```python
from build123d import *

# Parameters (mm, degrees)
SKETCH1_R           = 36.11499
BOSS_EXTRUDE1_DEPTH = 3.175
SKETCH2_R           = 9.525
BOSS_EXTRUDE3_DEPTH = 19.05
CHAMFER1_SIZE       = 4.7625
SKETCH5_R           = 15.875
BOSS_EXTRUDE4_DEPTH = 11.90625
BOSS_EXTRUDE5_DEPTH = 14.2875
CIRPATTERN1_COUNT   = 3
BOSS_EXTRUDE6_DEPTH = 14.2875
CIRPATTERN2_COUNT   = 6
SKETCH9_R           = 13.335
CUT_EXTRUDE1_DEPTH  = 11.90625
CHAMFER2_SIZE       = 0.762
CHAMFER3_SIZE       = 0.762


with BuildPart() as part:
    # Sketch1 → Boss-Extrude1 (new body)
    with BuildSketch(Plane(origin=(0, 0, 0), x_dir=(1, 0, 0), z_dir=(0, 1, 0))):
        with Locations(Location((0, 0, 0), (0, 0, 270))):
            Circle(SKETCH1_R)
    extrude(amount=BOSS_EXTRUDE1_DEPTH)

    # Sketch2 → Boss-Extrude3 (add)
    with BuildSketch(Plane(origin=(0, 3.175, 0), x_dir=(1, 0, 0), z_dir=(0, 1, 0))):
        with Locations(Location((0, 0, 0), (0, 0, 90))):
            Circle(SKETCH2_R)
    extrude(amount=BOSS_EXTRUDE3_DEPTH)

    # Chamfer1
    chamfer1_edges = [part.edges().sort_by_distance(p)[0] for p in [
        (0, 22.225, 9.525),
    ]]
    chamfer(chamfer1_edges, length=CHAMFER1_SIZE)

    # Sketch5 → Boss-Extrude4 (add)
    with BuildSketch(Plane.XZ):
        with Locations(Location((0, 0, 0), (0, 0, 270))):
            Circle(SKETCH5_R)
    extrude(amount=BOSS_EXTRUDE4_DEPTH)

    # Sketch6 → Boss-Extrude5 (add)
    with BuildSketch(Plane(origin=(0, 3.175, 0), x_dir=(1, 0, 0), z_dir=(0, 1, 0))):
        with BuildLine():
            Line((-1.5875, 36.080082406), (-1.5875, 9.391776656))
            ThreePointArc((-1.5875, 9.391776656), (0, 9.525), (1.5875, 9.391776656))
            Line((1.5875, 9.391776656), (1.5875, 33.101016708))
            ThreePointArc((1.5875, 33.101016708), (13.411669734, 30.303870682), (23.432855816, 23.432855816))
            Line((23.432855816, 23.432855816), (25.537154331, 25.537154331))
            ThreePointArc((25.537154331, 25.537154331), (13.083761644, 33.661664902), (-1.5875, 36.080082406))
        make_face()
    boss_extrude5 = extrude(amount=BOSS_EXTRUDE5_DEPTH)

    # CirPattern1: Boss-Extrude5 ×3 about axis
    cirpattern1_axis = Axis((0, 22.225, 0), (0, -1, 0))
    for i in range(1, CIRPATTERN1_COUNT):
        add(boss_extrude5.rotate(cirpattern1_axis, i * 360 / CIRPATTERN1_COUNT))

    # Sketch8 → Boss-Extrude6 (add)
    with BuildSketch(Plane(origin=(0, 3.175, 0), x_dir=(1, 0, 0), z_dir=(0, 1, 0))):
        with BuildLine():
            ThreePointArc((14.375330432, 18.734295362), (20.450378012, 11.80703125), (23.412040922, 3.082253661))
            Line((23.412040922, 3.082253661), (26.559878357, 3.496674321))
            ThreePointArc((26.559878357, 3.496674321), (23.200008669, 13.39453125), (16.308147969, 21.253192218))
            Line((16.308147969, 21.253192218), (14.375330432, 18.734295362))
        make_face()
    boss_extrude6 = extrude(amount=BOSS_EXTRUDE6_DEPTH)

    # CirPattern2: Boss-Extrude6 ×6 about axis
    cirpattern2_axis = Axis((0, 0, 0), (0, 1, 0))
    for i in range(1, CIRPATTERN2_COUNT):
        add(boss_extrude6.rotate(cirpattern2_axis, i * 360 / CIRPATTERN2_COUNT))

    # Sketch9 → Cut-Extrude1 (cut)
    with BuildSketch(Plane.XZ.offset(11.90625)):
        with Locations(Location((0, 0, 0), (0, 0, 270))):
            Circle(SKETCH9_R)
    extrude(amount=-CUT_EXTRUDE1_DEPTH, mode=Mode.SUBTRACT)

    # Chamfer2
    chamfer2_edges = [part.edges().sort_by_distance(p)[0] for p in [
        (0, 0, -36.11499),
    ]]
    chamfer(chamfer2_edges, length=CHAMFER2_SIZE)

    # Chamfer3
    chamfer3_edges = [part.edges().sort_by_distance(p)[0] for p in [
        (0, -11.90625, 15.875),
    ]]
    chamfer(chamfer3_edges, length=CHAMFER3_SIZE)


solid = part.part
```
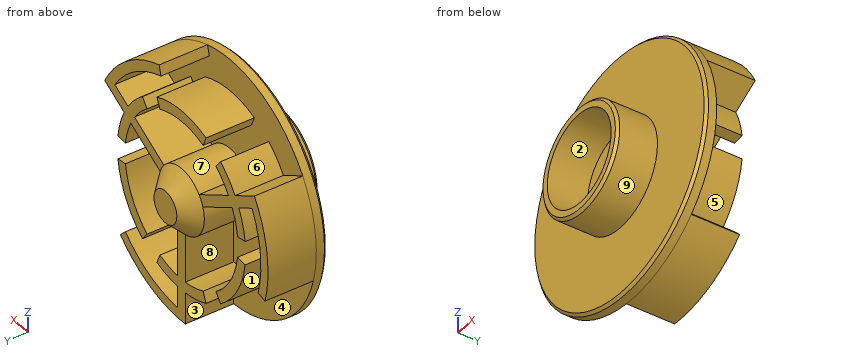
CAD build for the part. Positions are in the model's coordinates, mm. Face numbers are marked on the shaded views. A direction names the side the tool comes from. Round coordinates to 2 decimals unless told otherwise and drop trailing zeros. Order: outer loops, then holes, each group sorted by start corner. A loop starts at its lowest first (then second) coordinate and runs counter-clockwise, first axis right, second up.
Q1. Slice it at B-B (z = 0). Write the cut outline in (x, y) (1 decimal), and give its area (3 significant figures).
Q2. Which spindle directions (+Z, -Z, +X, -X, +Y, -Y) get a long thin tool onto all of the face, cutting with end or side? Do the marked faces 1, 2, 3, 4 and 5. Say none if no direction does.
Q3. Two-plate mould, pull along Z, no slides. Class the marked faces 6, 7, 8 and 9: pulls with the +Z half, pulls with the -Z half, needs draft (parallel to the pull), parting line crosses it, or undercut.
Q4. Slice it at C-C (y = 5). State how many separate pieces and enclosed holes the cut face has, and give its area (3 significant figures).
Q5. Drop flat-ended pins along their axis: pin 1 (8 mm diameter, centred on x = -10, z = -18, fed in from +Y); pin 2 (4.5 mm diameter, centred on y = 13, z = -33, fed in from -X); pin 3 (8 mm diameter, centred on y = -7.5, z = 26.5, fed in from +X); pin 4 (1.5 mm diameter, centred on y = 15, z = 5.5, fed in from -X). Give the stop position or say it passes through.
Q6. Slice it at A-A (x = 0). Write the cut outline in (y, z) (1 decimal).
Q7. Wall check: L1, parallel to X at y = -3.5, z = 0 (3 decimals); L2, parallel to X at y = 6.5, z = -6.5; L3, parallel to Z at x = 15.5, y = 8.5 (3 decimals). Give the ranges that are in metal, low to high.
Results below:
1. outline: (-36.1, 0.8) - (-35.4, 0) - (-15.9, 0) - (-15.9, -11.1) - (-15.1, -11.9) - (-13.3, -11.9) - (-13.3, 0) - (13.3, 0) - (13.3, -11.9) - (15.1, -11.9) - (15.9, -11.1) - (15.9, 0) - (35.4, 0) - (36.1, 0.8) - (36.1, 3.2) - (9.5, 3.2) - (9.5, 17.5) - (4.8, 22.2) - (-4.8, 22.2) - (-9.5, 17.5) - (-9.5, 3.2) - (-33.1, 3.2) - (-33.1, 17.5) - (-36.1, 17.5) - close
1. area: 671 mm2
2. face 1: -Z, +Y
2. face 2: -Y
2. face 3: -Z, -X, +Y
2. face 4: +Y
2. face 5: +X, +Y
3. face 6: pulls with the +Z half
3. face 7: undercut
3. face 8: undercut
3. face 9: parting line crosses it
4. separate pieces: 4
4. enclosed holes: 0
4. area: 1,110 mm2
5. pin 1: stops at y = 17.46
5. pin 2: stops at x = -1.59
5. pin 3: passes through
5. pin 4: stops at x = -35.8
6. outline: (-11.9, -15.1) - (-11.1, -15.9) - (0, -15.9) - (0, -35.4) - (0.8, -36.1) - (17.5, -36.1) - (17.5, -9.5) - (22.2, -4.8) - (22.2, 4.8) - (17.5, 9.5) - (3.2, 9.5) - (3.2, 23.6) - (17.5, 23.6) - (17.5, 26.8) - (3.2, 26.8) - (3.2, 36.1) - (0.8, 36.1) - (0, 35.4) - (0, 15.9) - (-11.1, 15.9) - (-11.9, 15.1) - (-11.9, 13.3) - (0, 13.3) - (0, -13.3) - (-11.9, -13.3) - close
7. L1: x = -15.875 to -13.335, 13.335 to 15.875
7. L2: x = -35.53 to -32.5, -25.99 to -22.7, -6.96 to 6.96, 22.7 to 25.99
7. L3: z = -32.62 to -29.291, -20.2 to -17.815, 7.116 to 10.782, 17.815 to 20.2, 29.291 to 32.62
